from build123d import *

# Parameters (mm, degrees)
F0_R     = 2.5527
F0_R_2   = 3.175
F0_R_3   = 14.2748
F0_R_4   = 12.7
F1_DEPTH = 6.35
F2_R     = 15.5575
F3_DEPTH = 1.6002


with BuildPart() as f1:
    # F0 (on Right) → F1 (new body)
    with BuildSketch(Plane.YZ):
        with BuildLine():
            Line((126.1410294417, 127), (25.4, 127))
            ThreePointArc((25.4, 127), (-10.5210244843, 112.1210244843), (-25.4, 76.2))
            Line((-25.4, 76.2), (0, 0))
            Line((0, 0), (12.7, 0))
            Line((12.7, 0), (25.4, 0))
            Line((25.4, 0), (101.6, 0))
            Line((101.6, 0), (127, 0))
            Line((127, 0), (144.6833077958, 103.5812))
            ThreePointArc((144.6833077958, 103.5812), (159.618637387, 134.4565300165), (126.1410294417, 127))
        make_face()
        with Locations((12.7, 12.7)):
            Circle(F0_R, mode=Mode.SUBTRACT)
        with Locations((12.7, 25.4)):
            Circle(F0_R, mode=Mode.SUBTRACT)
        with Locations((25.4, 12.7)):
            Circle(F0_R, mode=Mode.SUBTRACT)
        with Locations((25.4, 25.4)):
            Circle(F0_R, mode=Mode.SUBTRACT)
        with Locations((63.5, 63.5)):
            Circle(F0_R, mode=Mode.SUBTRACT)
        with Locations((88.9, 12.7)):
            Circle(F0_R, mode=Mode.SUBTRACT)
        with Locations((101.6, 12.7)):
            Circle(F0_R, mode=Mode.SUBTRACT)
        with Locations((88.9, 25.4)):
            Circle(F0_R, mode=Mode.SUBTRACT)
        with Locations((101.6, 25.4)):
            Circle(F0_R, mode=Mode.SUBTRACT)
        with Locations((88.9, 63.5)):
            Circle(F0_R_2, mode=Mode.SUBTRACT)
        with Locations((0, 76.2)):
            Circle(F0_R_3, mode=Mode.SUBTRACT)
        with Locations((38.1, 88.9)):
            Circle(F0_R, mode=Mode.SUBTRACT)
        with Locations((63.5, 88.9)):
            Circle(F0_R_4, mode=Mode.SUBTRACT)
        with Locations((38.1, 114.3)):
            Circle(F0_R_2, mode=Mode.SUBTRACT)
        with Locations((63.5, 114.3)):
            Circle(F0_R, mode=Mode.SUBTRACT)
        with Locations((88.9, 88.9)):
            Circle(F0_R, mode=Mode.SUBTRACT)
        with Locations((144.6833077958, 122.6312)):
            Circle(F0_R_3, mode=Mode.SUBTRACT)
    extrude(amount=F1_DEPTH)

    # F2 (on Right) → F3 (cut)
    with BuildSketch(Plane.YZ):
        with Locations((0, 76.2)):
            Circle(F2_R)
        with Locations((144.653, 122.6312)):
            Circle(F2_R)
    extrude(amount=F3_DEPTH, mode=Mode.SUBTRACT)


solid = f1.part
Part model, mm, in its own coordinate system. A direction names the side the tool comes from. Give positions to 0.01 mm unless a question says otherwise; leave off trailing zeros. Order: outer loops, then holes, each group sorted by start corner. A loop starts at its lowest first (then second) coordinate and runs counter-clockwise, first axis right, second up. Notation, with made-up numbers: (-6.5, 26) - (3.5, 26) arc R15 ccw to (3.5, 52) - close; hole circle Ø8 at (8, 37.25). An arc over 180 degrees is marked (long way). One line per question, with ' | ' between items.
1. Band-saw the part on A-A on y = 38.1. List the corners of the cut face in (x, z) (3 decimals).
Filled in:
outline: (0, 0) - (6.35, 0) - (6.35, 86.347) - (0, 86.347) - close; (0, 91.453) - (6.35, 91.453) - (6.35, 111.125) - (0, 111.125) - close; (0, 117.475) - (6.35, 117.475) - (6.35, 127) - (0, 127) - close
2. Band-saw the part on D-D on z = 25.4. List the corners of the cut face in (x, y), then the cut area to 3 significant figures.
Filled in:
outline: (0, -8.47) - (6.35, -8.47) - (6.35, 10.15) - (0, 10.15) - close; (0, 15.25) - (6.35, 15.25) - (6.35, 22.85) - (0, 22.85) - close; (0, 27.95) - (6.35, 27.95) - (6.35, 86.35) - (0, 86.35) - close; (0, 91.45) - (6.35, 91.45) - (6.35, 99.05) - (0, 99.05) - close; (0, 104.15) - (6.35, 104.15) - (6.35, 131.34) - (0, 131.34) - close | area: 758 mm²
3. Drop a flat-ended pin along its axis: P1, Ø18.5, axis at y = 144.65, z = 122.63, coming from the -X side. Give the stop position or say it passes through.
Filled in:
P1: through
4. Band-saw the part on B-B on x = 3.5. Give the number of separate pieces and of enclosed holes in the cut face, then the cut area to 3 significant figures.
Filled in:
separate pieces: 1 | enclosed holes: 17 | area: 17,800 mm²
5. Drill centre lines: probe 1 along Z at (x, y) = (1.75, 88.9) (3 decimals); probe 2 along Z at (x, y) = (2.75, 101.6); probe 3 along Z at (x, y) = (1.5, 63.5). Where is each one in solid material? Low to high.
Filled in:
probe 1: 0 to 10.147, 15.253 to 22.847, 27.953 to 60.325, 66.675 to 86.347, 91.453 to 127 | probe 2: 0 to 10.15, 15.25 to 22.85, 27.95 to 127 | probe 3: 0 to 60.95, 66.05 to 76.2, 101.6 to 111.75, 116.85 to 127
6. Which spindle directions (+Z, -Z, +X, -X, +Y, -Y) get a long thin tool onto all of the face, cutting with end or side? Do faces 1 (the face through (1.6, 13, 69)), 2 (the face through (0, 68, 72)). Say none if no direction does.
Filled in:
face 1: -X | face 2: +Z, -Z, -X, +Y, -Y
7. Band-saw the part on C-C on y = 132.5. List the corners of the cut face in (x, z).
Filled in:
outline: (0, 32.22) - (6.35, 32.22) - (6.35, 115.19) - (1.6, 115.19) - (1.6, 112.92) - (0, 112.92) - close; (0, 132.34) - (1.6, 132.34) - (1.6, 130.07) - (6.35, 130.07) - (6.35, 137.28) - (0, 137.28) - close
8. Pull direction Z, two halves, no side cores. Call faces 3 (the face through (3, 76, 127)), 4 (the face through (3.13, 135.72, 51.07)), 5 (the face through (3.131, 15.058, 11.722)): +Z half, -Z half, draft (parallel to the pull), parting line (faces both ways), or undercut.
Filled in:
face 3: +Z half | face 4: -Z half | face 5: undercut
